Check sheet for the modelled part. Datum: model origin and axes. Units: mm. Round coordinates to 2 decimals unless told otherwise and drop trailing zeros. Write each loop counter-clockwise with the first axis right and the second up, starting at its lowest first coordinate (ties: lowest second). Pieces come first, ordered by that corner, then holes.
Item 1: Material ranges on line 1 along Y through (x, z) = (22, -0.2); line 2 along X through (y, z) = (6.75, -0.4); line 3 along X through (y, z) = (-1.25, -0.55), recorded low to high.
Item 2: Section check B-B, the plane x = 6. Record the cut outline in (y, z).
Item 3: Section check A-A, the plane y = 11.75. Record the cut outline in (x, z), plus the area to 3 significant figures.
Item 4: Depth check by flat-ended pin: pin 1 (4.5 mm diameter, centred on x = 10.91, y = -1.57, fed in from -Z); pin 2 (2 mm diameter, centred on x = 16.5, y = 8.5, fed in from +Z). Enter the tip coordinate at first touch or a pass-through.
from build123d import *

# Parameters (mm, degrees)
SKETCH1_R               = 34.867744869
BASE_FLANGE1_DEPTH      = 0.7366
CUT_EXTRUDE1_DEPTH      = 166.090690723
CUT_EXTRUDE1_DEPTH_BACK = 166.090690723
SKETCH2_R               = 180.553154812
CUT_EXTRUDE2_DEPTH      = 143.907778027
CUT_EXTRUDE2_DEPTH_BACK = 143.907778027


# Sheet-metal steps are written as plain solids
with BuildPart() as part:
    # Sketch1 → Base-Flange1 (new body)
    with BuildSketch(Plane.XY):
        Circle(SKETCH1_R)
    extrude(amount=-BASE_FLANGE1_DEPTH)

    # Sketch2 → Cut-Extrude1 (cut, two sides: drawn at the far end of the back side and taken through both)
    with BuildSketch(Plane(origin=(-59.555266985, -54.618905297, 100.906749206), x_dir=(-1, 0, 0), z_dir=(0, 0, -1)).offset(-CUT_EXTRUDE1_DEPTH_BACK)):
        with Locations((-70.46331512, 53.044531114)):
            Circle(SKETCH2_R)
        with BuildLine():
            Line((-81.344420416, 48.08529911), (-81.147360116, 48.260073924))
            ThreePointArc((-81.147360116, 48.260073924), (-80.592208079, 48.791271643), (-80.078779721, 49.362897501))
            ThreePointArc((-80.078779721, 49.362897501), (-79.183035074, 52.245324657), (-80.587831747, 54.91689556))
            ThreePointArc((-80.587831747, 54.91689556), (-81.196617582, 55.385664809), (-81.839082773, 55.807094848))
            Line((-81.839082773, 55.807094848), (-82.06463088, 55.943135463))
            ThreePointArc((-82.06463088, 55.943135463), (-83.339743584, 56.936582022), (-84.344361609, 58.202911795))
            ThreePointArc((-84.344361609, 58.202911795), (-83.910146998, 59.247357512), (-83.397480034, 60.255614309))
            ThreePointArc((-83.397480034, 60.255614309), (-81.782081355, 60.31336879), (-80.198688666, 59.98822872))
            Line((-80.198688666, 59.98822872), (-79.948799088, 59.904956901))
            ThreePointArc((-79.948799088, 59.904956901), (-79.21119235, 59.689779993), (-78.459435657, 59.530950921))
            ThreePointArc((-78.459435657, 59.530950921), (-75.515308192, 60.196426879), (-73.904058259, 62.748801937))
            ThreePointArc((-73.904058259, 62.748801937), (-73.802485098, 63.51041056), (-73.758748573, 64.277516756))
            Line((-73.758748573, 64.277516756), (-73.753707998, 64.540867454))
            ThreePointArc((-73.753707998, 64.540867454), (-73.530914393, 66.141870727), (-72.936549652, 67.645060345))
            ThreePointArc((-72.936549652, 67.645060345), (-71.814925823, 67.79124232), (-70.685416342, 67.851388104))
            ThreePointArc((-70.685416342, 67.851388104), (-69.827700155, 66.481289051), (-69.317583371, 64.947460723))
            Line((-69.317583371, 64.947460723), (-69.264754091, 64.689414091))
            ThreePointArc((-69.264754091, 64.689414091), (-69.082299391, 63.943039464), (-68.843971056, 63.212584534))
            ThreePointArc((-68.843971056, 63.212584534), (-66.795588238, 60.995633336), (-63.779541631, 60.876437491))
            ThreePointArc((-63.779541631, 60.876437491), (-63.069182636, 61.169276865), (-62.38298092, 61.514953022))
            Line((-62.38298092, 61.514953022), (-62.152392238, 61.642263104))
            ThreePointArc((-62.152392238, 61.642263104), (-60.654485929, 62.249819819), (-59.055503163, 62.486679664))
            ThreePointArc((-59.055503163, 62.486679664), (-58.368093945, 61.588415921), (-57.751251427, 60.640304909))
            ThreePointArc((-57.751251427, 60.640304909), (-58.508933919, 59.212451375), (-59.582209824, 58.003763118))
            Line((-59.582209824, 58.003763118), (-59.779270124, 57.828988304))
            ThreePointArc((-59.779270124, 57.828988304), (-60.334422161, 57.297790585), (-60.847850519, 56.726164727))
            ThreePointArc((-60.847850519, 56.726164727), (-61.743595166, 53.843737571), (-60.338798493, 51.172166668))
            ThreePointArc((-60.338798493, 51.172166668), (-59.730012659, 50.703397419), (-59.087547467, 50.28196738))
            Line((-59.087547467, 50.28196738), (-58.861999361, 50.145926765))
            ThreePointArc((-58.861999361, 50.145926765), (-57.586886657, 49.152480206), (-56.582268631, 47.886150433))
            ThreePointArc((-56.582268631, 47.886150433), (-57.016483242, 46.841704716), (-57.529150206, 45.833447919))
            ThreePointArc((-57.529150206, 45.833447919), (-59.144548885, 45.775693438), (-60.727941574, 46.100833508))
            Line((-60.727941574, 46.100833508), (-60.977831152, 46.184105327))
            ThreePointArc((-60.977831152, 46.184105327), (-61.71543789, 46.399282235), (-62.467194583, 46.558111307))
            ThreePointArc((-62.467194583, 46.558111307), (-65.411322049, 45.892635349), (-67.022571982, 43.340260291))
            ThreePointArc((-67.022571982, 43.340260291), (-67.124145142, 42.578651669), (-67.167881667, 41.811545472))
            Line((-67.167881667, 41.811545472), (-67.172922242, 41.548194774))
            ThreePointArc((-67.172922242, 41.548194774), (-67.395715847, 39.947191501), (-67.990080588, 38.444001883))
            ThreePointArc((-67.990080588, 38.444001883), (-69.111704417, 38.297819908), (-70.241213899, 38.237674124))
            ThreePointArc((-70.241213899, 38.237674124), (-71.098930085, 39.607773177), (-71.60904687, 41.141601505))
            Line((-71.60904687, 41.141601505), (-71.661876149, 41.399648137))
            ThreePointArc((-71.661876149, 41.399648137), (-71.844330849, 42.146022764), (-72.082659185, 42.876477694))
            ThreePointArc((-72.082659185, 42.876477694), (-74.131042002, 45.093428892), (-77.147088609, 45.212624737))
            ThreePointArc((-77.147088609, 45.212624737), (-77.857447604, 44.919785363), (-78.54364932, 44.574109206))
            Line((-78.54364932, 44.574109206), (-78.774238002, 44.446799124))
            ThreePointArc((-78.774238002, 44.446799124), (-80.272144311, 43.839242409), (-81.871127077, 43.602382564))
            ThreePointArc((-81.871127077, 43.602382564), (-82.558536295, 44.500646307), (-83.175378813, 45.448757319))
            ThreePointArc((-83.175378813, 45.448757319), (-82.417696321, 46.876610853), (-81.344420416, 48.08529911))
        make_face(mode=Mode.SUBTRACT)
    extrude(amount=CUT_EXTRUDE1_DEPTH + CUT_EXTRUDE1_DEPTH_BACK, mode=Mode.SUBTRACT)

    # Sketch3 → Cut-Extrude2 (cut, two sides: drawn at the far end of the back side and taken through both)
    with BuildSketch(Plane(origin=(-59.555266985, -54.618905297, 92.56319002), x_dir=(-1, 0, 0), z_dir=(0, 0, -1)).offset(-CUT_EXTRUDE2_DEPTH_BACK)):
        with BuildLine():
            Line((-69.183385772, 51.044048454), (-68.447999148, 54.300975121))
            ThreePointArc((-68.447999148, 54.300975121), (-72.779897357, 53.567595882), (-69.183385772, 51.044048454))
        make_face()
    extrude(amount=CUT_EXTRUDE2_DEPTH + CUT_EXTRUDE2_DEPTH_BACK, mode=Mode.SUBTRACT)


solid = part.part
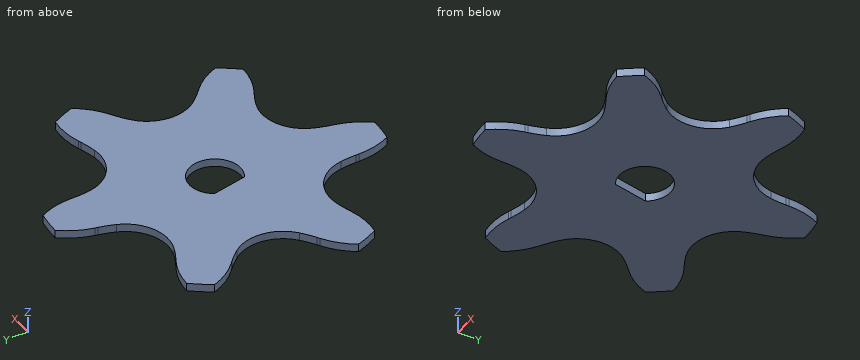
Values found:
1. line 1: y = -11 to -6.73, 1.01 to 5.67
1. line 2: x = -1.34 to 3.1, 7.88 to 14.87
1. line 3: x = 2.12 to 9.1, 13.26 to 19.9
2. outline: (-8.83, -0.74) - (6.04, -0.74) - (6.04, 0) - (-8.83, 0) - close
3. outline: (10.22, -0.74) - (13.91, -0.74) - (13.91, 0) - (10.22, 0) - close
3. area: 2.72 mm2
4. pin 1: stops at z = -0.74
4. pin 2: passes through
